Drawing for the job (mm, zero at the part's lowest x, y, z). A direction names the side the tool comes from. Give positions to 0.01 mm unless a question says otherwise; leave off trailing zeros. Order: outer loops, then holes, each group sorted by start corner. A loop starts at its lowest first (then second) coordinate and runs counter-clockwise, first axis right, second up. Notation, with made-up numbers: (61.25, 38) - (71.25, 38) arc R14 cw to (71.25, 52) - close; hole circle Ø4 at (81.25, -1.5). An arc over 180 degrees is marked (long way). Use CSV: the item, a comma, the result in double quotes. Start each with the question number.
(1) Drop flat-ended pins along their axis: pin 1 Ø10 at (x, y) = (101, 46) entering from -Z; pin 2 Ø8 at (x, y) = (66, 101.5) entering from +Z. Give the stop position or say it passes through.
(2) Band-saw the part on B-B, the plane x = 60. Give the cut face in (y, z), then the cut area to 3 significant figures.
(3) Probe L1, parallel to X at y = 182, z = 26; L2, parallel to Y at x = 55.5, z = 39; L3, parallel to Z at x = 91.5, y = 26. List the from-to ranges inside material, lowest first.
(4) Tool access for the marked faces 1 and 2: list every direction of +Z, -Z, +X, -X, +Y, -Y with a clear straight run to the whole face (end or side of a thin tool).
(5) Band-saw the part on A-A, the plane z = 20. Give the cut face in (x, y).
(6) Band-saw the part on C-C, the plane y = 83. Give the cut face in (x, z).
(7) Pull direction Y, two halves, no side cores. Call the marked faces 3, 4 and 5: +Y half, -Y half, draft (parallel to the pull), parting line (faces both ways), or undercut.
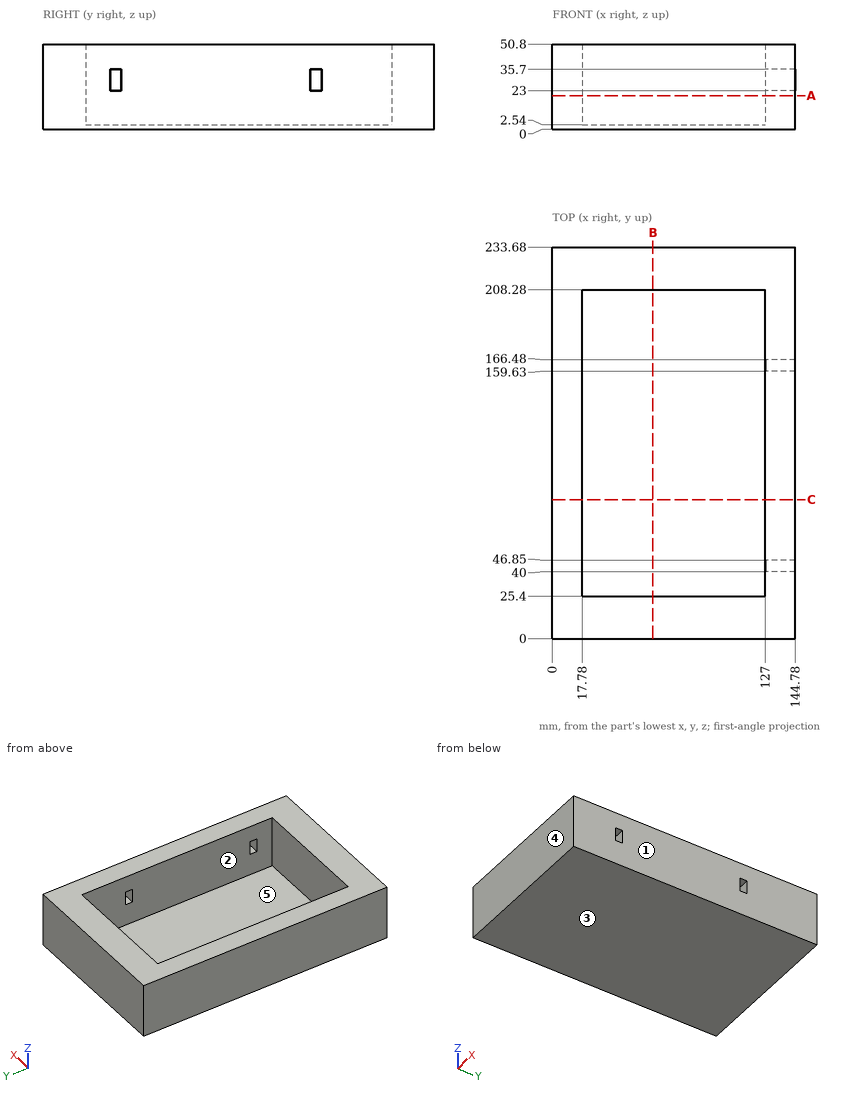
Answer block:
1,pin 1,"stops at z = 0"
1,pin 2,"stops at z = 2.54"
2,outline,"(0, 0) - (233.68, 0) - (233.68, 50.8) - (208.28, 50.8) - (208.28, 2.54) - (25.4, 2.54) - (25.4, 50.8) - (0, 50.8) - close"
2,area,"3,050 mm2"
3,L1,"x = 0 to 17.78, 127 to 144.78"
3,L2,"y = 0 to 25.4, 208.28 to 233.68"
3,L3,"z = 0 to 2.54"
4,face 1,"+Z, -Z, +X, +Y, -Y"
4,face 2,"+Z"
5,outline,"(0, 0) - (144.78, 0) - (144.78, 233.68) - (0, 233.68) - close; hole (17.78, 25.4) - (127, 25.4) - (127, 208.28) - (17.78, 208.28) - close"
6,outline,"(0, 0) - (144.78, 0) - (144.78, 50.8) - (127, 50.8) - (127, 2.54) - (17.78, 2.54) - (17.78, 50.8) - (0, 50.8) - close"
7,face 3,"draft"
7,face 4,"-Y half"
7,face 5,"undercut"
